For this review, take the finished solid that the model builds, in its own axes (mm). A direction names the side the tool comes from. Round coordinates to 2 decimals unless told otherwise and drop trailing zeros. Order: outer loops, then holes, each group sorted by start corner. A loop starts at its lowest first (then second) coordinate and runs counter-clockwise, first axis right, second up. Notation, with made-up numbers: M 85.5,1 L 89.5,1 A20 cw 89.5,12 Z; hole C 61,82 d9. An arc over 180 degrees is marked long. Put each result on its own line as item: value.
Autodesk Inventor part; units mm, degrees
ref_plane "Work Plane7" through (0, 79.375, 0) normal (0, 1, 0) x (-1, 0, 0)
ref_plane "YZ Plane" through (0, 0, 0) normal (1, 0, 0) x (0, 1, 0)
ref_plane "XY Plane" through (0, 0, 0) normal (0, 0, 1) x (1, 0, 0)
sketch "Sketch8" plane through (0, 0, 0) normal (0, 0, 1) x (1, 0, 0)
  arc A0 (76.1338, 3.175) -> (-76.1338, 3.175) centre (0, 0) ccw
  arc A1 (81.9986, 9.525) -> (-81.9986, 9.525) centre (0, 0) ccw
  line L0 (-82.4889, 3.175) -> (-101.5389, 3.175)
  line L1 (-101.5389, 3.175) -> (-101.5389, 9.525)
  line L2 (-101.5389, 9.525) -> (-81.9986, 9.525)
  line L3 (0, 0) -> (0, 82.55) construction
  line L4 (-82.4889, 3.175) -> (-76.1338, 3.175)
  line L5 (82.4889, 3.175) -> (101.5389, 3.175)
  line L6 (101.5389, 3.175) -> (101.5389, 9.525)
  line L7 (101.5389, 9.525) -> (81.9986, 9.525)
  line L8 (82.4889, 3.175) -> (76.1338, 3.175)
  dimension "d52" = 152.4
  dimension "d53" = 6.35
  dimension "d54" = 19.05
  dimension "d55" = 3.175
  dimension "d56" = 6.35
extrude "Extrusion5" add sketch "Sketch8" along normal mid plane 76.2
sketch "Sketch9" plane through (-101.5389, 9.525, 38.1) normal (0, 1, 0) x (1, 0, 0)
  line L0 (19.5403, 0) -> (0, 0) construction
  line L1 (9.7701, 0) -> (9.7701, 76.2) construction
  line L2 (25.4051, 76.2) -> (0, 76.2) construction
  line L3 (9.7701, 25.4) -> (9.7701, 101.6) construction
  line L4 (9.7701, 50.8) -> (9.7701, 127) construction
  point P0 (101.5389, 38.1)
  point P1 (9.7701, 12.7)
  point P2 (9.7701, 38.1)
  point P3 (9.7701, 63.5)
  dimension "d59" = 12.7
  dimension "d62" = 25.4
hole "Hole3" at (-91.7688, 9.525, 25.4) at (-91.7688, 9.525, 0) at (-91.7688, 9.525, -25.4) direction (0, -1, 0) diameter 6.7564 end through all
mirror "Mirror3" about plane through (0, 0, 0) normal (1, 0, 0) of "Hole3"
ref_plane "Work Plane7" through (0, 79.375, 0) normal (0, 1, 0) x (-1, 0, 0)
sketch "Sketch20" plane through (0, 79.375, 0) normal (0, 1, 0) x (-1, 0, 0)
  circle A0 centre (0, 0) radius 9.525
  dimension "d101" = 19.05
extrude "Extrusion11" add sketch "Sketch20" along normal blind 50.8
sketch "Sketch21" plane through (0, 130.175, 0) normal (0, 1, 0) x (1, 0, 0)
  arc A0 (1.5875, 9.3918) -> (-1.5875, 9.3918) centre (0, 0) ccw
  circle A1 centre (0, 0) radius 9.525
  line L0 (-1.5875, 9.3918) -> (-1.5875, 6.35)
  line L1 (-1.5875, 6.35) -> (1.5875, 6.35)
  line L2 (1.5875, 6.35) -> (1.5875, 9.3918)
  dimension "d106" = 3.175
  dimension "d107" = 3.175
extrude "Extrusion12" cut sketch "Sketch21" against normal blind 25.4 contours L2 L1 L0 A0
pattern_circular "Circular Pattern3" count 6 over 360 about axis through (0, -10, 0) along (0, 1, 0) of "Extrusion12"
properties part number "tubeBracket" material "ABS Plastic"
(1) Add section A-A on z = 25.4. Give the boundary of the cut face in (x, y) (3 decimals), then the cut area to 3 significant figures.
A:
outline: M -101.539,3.175 L -95.147,3.175 L -95.147,9.525 L -101.539,9.525 Z; M -88.391,3.175 L -76.134,3.175 A76.2 cw 76.134,3.175 L 88.391,3.175 L 88.391,9.525 L 81.999,9.525 A82.55 ccw -81.999,9.525 L -88.391,9.525 Z; M 95.147,3.175 L 101.539,3.175 L 101.539,9.525 L 95.147,9.525 Z
area: 1,700 mm2
(2) Add section B-B on y = 60. Give the boundary of the cut face in (x, z).
A:
outline: M -56.7,-38.1 L -46.97,-38.1 L -46.97,38.1 L -56.7,38.1 Z; M 46.97,-38.1 L 56.7,-38.1 L 56.7,38.1 L 46.97,38.1 Z
(3) To check wall thickness, follow L1, parallel to X at y = 4, z = 0; L2, parallel to X at y = 5, z = 25; L3, parallel to X at y = 63, z = 27.5. State the ranges of each line that lie inside material, in increasing order.
A:
L1: x = -101.54 to -95.15, -88.39 to -76.09, 76.09 to 88.39, 95.15 to 101.54
L2: x = -101.54 to -95.12, -88.41 to -76.04, 76.04 to 88.41, 95.12 to 101.54
L3: x = -53.34 to -42.87, 42.87 to 53.34
(4) Draft analysis for pull direction X (two halves, no side actions). For faces 6 (the face through (7, 104.775, 4)), 7 (the face through (-89.71, 6.31, -28.08)), 8 (the face through (-101.539, 6, -1)), 9 (the face through (-16, 75, 38.1)), state which applies: released by +X, released by -X, zero draft, split by the parting line, or undercut.
A:
face 6: undercut
face 7: undercut
face 8: released by -X
face 9: zero draft
(5) Add section D-D on x = -21.5. Give the boundary of the cut face in (y, z).
A:
outline: M 73.1,-38.1 L 79.7,-38.1 L 79.7,38.1 L 73.1,38.1 Z
(6) Add section C-C on y = 44. Give the boundary of the cut face in (x, z).
A:
outline: M -69.85,-38.1 L -62.21,-38.1 L -62.21,38.1 L -69.85,38.1 Z; M 62.21,-38.1 L 69.85,-38.1 L 69.85,38.1 L 62.21,38.1 Z
(7) For faces 1 (the face through (101.539, 6, -1)), 2 (the face through (-96, 9.525, -1)), 3 (the face through (-88.772, 6.306, 1.559)), 4 (the face through (-9.085, 105.749, -2.861)), 5 (the face through (96, 9.525, -1)), list the 3-axis set-ups (+Z, -Z, +X, -X, +Y, -Y) from which the entire face can be reached by the end or side of a thin tool; tool diameter is ignored.
A:
face 1: +Z, -Z, +X, +Y, -Y
face 2: +Z, -Z, -X, +Y
face 3: +Y, -Y
face 4: +Y
face 5: +Z, -Z, +X, +Y
(8) Insertion check: pin 1 Ø0.9 at (y, z) = (114.5, 8.5) entering from +X; pin 2 Ø1 at (x, z) = (-41, -30) entering from +Y; pin 3 Ø6 at (x, z) = (87, 12.5) entering from +Y (3 decimals); pin 4 Ø4 at (x, z) = (-91.77, 0) entering from +Y. Each pin has a flat end and moves straight along its axis. Give the tip position at first contact, or say it passes through.
A:
pin 1: stops at x = 5.09
pin 2: stops at y = 71.93
pin 3: stops at y = 9.525
pin 4: passes through
